from build123d import *

# Parameters (mm, degrees)
BOSS_EXTRUDE1_DEPTH = 220
CUT_EXTRUDE1_REACH  = 245.655
SKETCH2_R           = 2
SKETCH3_R           = 20
CUT_EXTRUDE2_DEPTH  = 220


with BuildPart() as part:
    # Sketch1 → Boss-Extrude1 (new body)
    with BuildSketch(Plane.XY):
        Polygon((0, -51.046601942), (0, 50.553398058), (25.4, 50.553398058), (25.4, 47.378398058), (3.175, 47.378398058), (3.175, -47.871601942), (25.4, -47.871601942), (25.4, -51.046601942), align=None)
    extrude(amount=BOSS_EXTRUDE1_DEPTH)

    # Cut-Extrude1: up to this face of the body (flat: up to its plane)
    cut_extrude1_end = Plane(part.part.faces().sort_by_distance((12.7, -51.046601942, 110))[0])
    # Sketch2 → Cut-Extrude1 (cut, up to the picked face)
    with BuildSketch(Plane(origin=(0, 50.553398058, 0), x_dir=(1, 0, 0), z_dir=(0, 1, 0)), mode=Mode.PRIVATE) as cut_extrude1_sk1:
        with Locations(Location((12.7, -110, 0), (0, 0, 270))):
            Circle(SKETCH2_R)
    cut_extrude1_tool1 = split(extrude(cut_extrude1_sk1.sketch, amount=-CUT_EXTRUDE1_REACH, mode=Mode.PRIVATE), bisect_by=cut_extrude1_end, keep=Keep.BOTH, mode=Mode.PRIVATE)
    # Sketch2 → Cut-Extrude1 (cut, up to the picked face)
    with BuildSketch(Plane(origin=(0, 50.553398058, 0), x_dir=(1, 0, 0), z_dir=(0, 1, 0)), mode=Mode.PRIVATE) as cut_extrude1_sk2:
        with Locations(Location((12.7, -80, 0), (0, 0, 270))):
            Circle(SKETCH2_R)
    cut_extrude1_tool2 = split(extrude(cut_extrude1_sk2.sketch, amount=-CUT_EXTRUDE1_REACH, mode=Mode.PRIVATE), bisect_by=cut_extrude1_end, keep=Keep.BOTH, mode=Mode.PRIVATE)
    # Sketch2 → Cut-Extrude1 (cut, up to the picked face)
    with BuildSketch(Plane(origin=(0, 50.553398058, 0), x_dir=(1, 0, 0), z_dir=(0, 1, 0)), mode=Mode.PRIVATE) as cut_extrude1_sk3:
        with Locations(Location((12.7, -50, 0), (0, 0, 270))):
            Circle(SKETCH2_R)
    cut_extrude1_tool3 = split(extrude(cut_extrude1_sk3.sketch, amount=-CUT_EXTRUDE1_REACH, mode=Mode.PRIVATE), bisect_by=cut_extrude1_end, keep=Keep.BOTH, mode=Mode.PRIVATE)
    # Sketch2 → Cut-Extrude1 (cut, up to the picked face)
    with BuildSketch(Plane(origin=(0, 50.553398058, 0), x_dir=(1, 0, 0), z_dir=(0, 1, 0)), mode=Mode.PRIVATE) as cut_extrude1_sk4:
        with Locations(Location((12.7, -20, 0), (0, 0, 270))):
            Circle(SKETCH2_R)
    cut_extrude1_tool4 = split(extrude(cut_extrude1_sk4.sketch, amount=-CUT_EXTRUDE1_REACH, mode=Mode.PRIVATE), bisect_by=cut_extrude1_end, keep=Keep.BOTH, mode=Mode.PRIVATE)
    # Sketch2 → Cut-Extrude1 (cut, up to the picked face)
    with BuildSketch(Plane(origin=(0, 50.553398058, 0), x_dir=(1, 0, 0), z_dir=(0, 1, 0)), mode=Mode.PRIVATE) as cut_extrude1_sk5:
        with Locations(Location((12.7, -140, 0), (0, 0, 270))):
            Circle(SKETCH2_R)
    cut_extrude1_tool5 = split(extrude(cut_extrude1_sk5.sketch, amount=-CUT_EXTRUDE1_REACH, mode=Mode.PRIVATE), bisect_by=cut_extrude1_end, keep=Keep.BOTH, mode=Mode.PRIVATE)
    # Sketch2 → Cut-Extrude1 (cut, up to the picked face)
    with BuildSketch(Plane(origin=(0, 50.553398058, 0), x_dir=(1, 0, 0), z_dir=(0, 1, 0)), mode=Mode.PRIVATE) as cut_extrude1_sk6:
        with Locations(Location((12.7, -170, 0), (0, 0, 270))):
            Circle(SKETCH2_R)
    cut_extrude1_tool6 = split(extrude(cut_extrude1_sk6.sketch, amount=-CUT_EXTRUDE1_REACH, mode=Mode.PRIVATE), bisect_by=cut_extrude1_end, keep=Keep.BOTH, mode=Mode.PRIVATE)
    # Sketch2 → Cut-Extrude1 (cut, up to the picked face)
    with BuildSketch(Plane(origin=(0, 50.553398058, 0), x_dir=(1, 0, 0), z_dir=(0, 1, 0)), mode=Mode.PRIVATE) as cut_extrude1_sk7:
        with Locations(Location((12.7, -200, 0), (0, 0, 270))):
            Circle(SKETCH2_R)
    cut_extrude1_tool7 = split(extrude(cut_extrude1_sk7.sketch, amount=-CUT_EXTRUDE1_REACH, mode=Mode.PRIVATE), bisect_by=cut_extrude1_end, keep=Keep.BOTH, mode=Mode.PRIVATE)
    add(cut_extrude1_tool1.solids().sort_by(Axis((12.7, 50.553398, 110), (0, -1, 0)))[0], mode=Mode.SUBTRACT)
    add(cut_extrude1_tool2.solids().sort_by(Axis((12.7, 50.553398, 80), (0, -1, 0)))[0], mode=Mode.SUBTRACT)
    add(cut_extrude1_tool3.solids().sort_by(Axis((12.7, 50.553398, 50), (0, -1, 0)))[0], mode=Mode.SUBTRACT)
    add(cut_extrude1_tool4.solids().sort_by(Axis((12.7, 50.553398, 20), (0, -1, 0)))[0], mode=Mode.SUBTRACT)
    add(cut_extrude1_tool5.solids().sort_by(Axis((12.7, 50.553398, 140), (0, -1, 0)))[0], mode=Mode.SUBTRACT)
    add(cut_extrude1_tool6.solids().sort_by(Axis((12.7, 50.553398, 170), (0, -1, 0)))[0], mode=Mode.SUBTRACT)
    add(cut_extrude1_tool7.solids().sort_by(Axis((12.7, 50.553398, 200), (0, -1, 0)))[0], mode=Mode.SUBTRACT)

    # Sketch3 → Cut-Extrude2 (cut)
    with BuildSketch(Plane.ZY):
        with Locations((110, 0)):
            Circle(SKETCH3_R)
    extrude(amount=-CUT_EXTRUDE2_DEPTH, mode=Mode.SUBTRACT)


solid = part.part
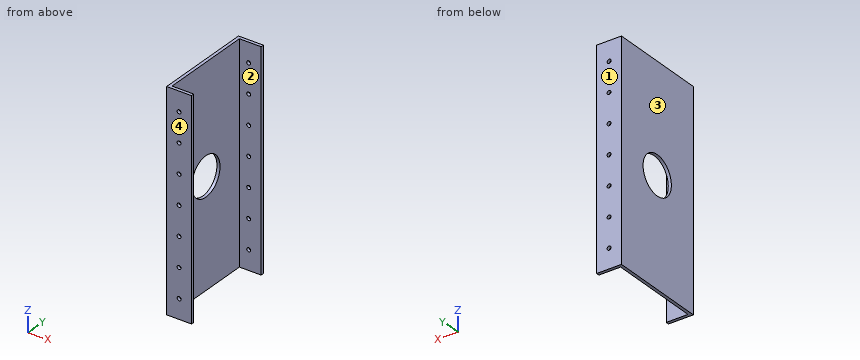
CAD build for the part. Positions are in the model's coordinates, mm. Face numbers are marked on the shaded views. Round coordinates to 2 decimals unless told otherwise and drop trailing zeros. Loops run counter-clockwise (first coordinate to the right, second up) from the corner with the lowest first, then second, coordinate; pieces in that order, holes last. Notation, with made-up numbers: (-37.5, -26) - (-20.5, -26) arc R27 ccw to (-20.5, -10) - close; hole circle Ø10 at (88, 80). An arc over 180 degrees is marked (long way). Put each result on its own line as item: value.
1. Slice it at D-D on z = 110. List the corners of the cut face in (x, y) (3 decimals).
Geometry check:
outline: (0, -51.047) - (10.7, -51.047) - (10.7, -47.872) - (3.175, -47.872) - (3.175, -20) - (0, -20) - close; (0, 20) - (3.175, 20) - (3.175, 47.378) - (10.7, 47.378) - (10.7, 50.553) - (0, 50.553) - close; (14.7, -51.047) - (25.4, -51.047) - (25.4, -47.872) - (14.7, -47.872) - close; (14.7, 47.378) - (25.4, 47.378) - (25.4, 50.553) - (14.7, 50.553) - close
2. Slice it at C-C on x = 19.25. List the corners of the cut face in (y, z).
Geometry check:
outline: (-51.05, 0) - (-47.87, 0) - (-47.87, 220) - (-51.05, 220) - close; (47.38, 0) - (50.55, 0) - (50.55, 220) - (47.38, 220) - close
3. Pin check, flat tips, straight feed: P1, Ø3, axis at x = 12.7, z = 170, coming from the +Y side; P2, Ø3, axis at y = 38.5, z = 135, coming from the +X side (3 decimals). Stop position of each tip, or through.
Geometry check:
P1: through
P2: x = 3.175
4. Wall check: line 1 (Y direction, x = 12.5, z = 160); line 2 (X direction, y = 48.7, z = 200); line 3 (X direction, y = -28.5, z = 200) (3 decimals). Give the ranges that are in metal, low to high.
Geometry check:
line 1: -51.05 to -47.87, 47.38 to 50.55
line 2: 0 to 10.7, 14.7 to 25.4
line 3: 0 to 3.175
5. Slice it at A-A on z = 200. List the corners of the cut face in (x, y) (3 decimals), and give its area (3 significant figures).
Geometry check:
outline: (0, -51.047) - (10.7, -51.047) - (10.7, -47.872) - (3.175, -47.872) - (3.175, 47.378) - (10.7, 47.378) - (10.7, 50.553) - (0, 50.553) - close; (14.7, -51.047) - (25.4, -51.047) - (25.4, -47.872) - (14.7, -47.872) - close; (14.7, 47.378) - (25.4, 47.378) - (25.4, 50.553) - (14.7, 50.553) - close
area: 438 mm²
6. Two-plate mould, pull along Y, no slides. Class the marked faces 1, 2, 3 and 4: released by +Y, released by -Y, zero draft, split by the parting line, or undercut.
Geometry check:
face 1: released by +Y
face 2: undercut
face 3: zero draft
face 4: released by -Y
7. Slice it at B-B on y = -5.5. List the corners of the cut face in (x, z) (3 decimals), and give its area (3 significant figures).
Geometry check:
outline: (0, 0) - (3.175, 0) - (3.175, 90.771) - (0, 90.771) - close; (0, 129.229) - (3.175, 129.229) - (3.175, 220) - (0, 220) - close
area: 576 mm²
